```python
from build123d import *

# Parameters (mm, degrees)
SKETCH2_W           = 200
SKETCH2_H           = 150
SKETCH2_W_2         = 190
SKETCH2_H_2         = 140
BOSS_EXTRUDE1_DEPTH = 1800
SKETCH5_R           = 2.5
CUT_EXTRUDE3_DEPTH  = 10
SKETCH6_R           = 5
SKETCH6_R_2         = 2
CUT_EXTRUDE4_DEPTH  = 5


with BuildPart() as part:
    # Sketch2 → Boss-Extrude1 (new body)
    with BuildSketch(Plane.XY):
        Rectangle(SKETCH2_W, SKETCH2_H)
        Rectangle(SKETCH2_W_2, SKETCH2_H_2, mode=Mode.SUBTRACT)
    extrude(amount=BOSS_EXTRUDE1_DEPTH)

    # Sketch5 → Cut-Extrude3 (cut)
    with BuildSketch(Plane(origin=(0, 75, 0), x_dir=(1, 0, 0), z_dir=(0, 1, 0))):
        with Locations((-32.7, -360)):
            Circle(SKETCH5_R)
        with Locations((-32.7, -480)):
            Circle(SKETCH5_R)
        with Locations((-32.7, -600)):
            Circle(SKETCH5_R)
        with Locations((-32.7, -720)):
            Circle(SKETCH5_R)
        with Locations((-32.7, -840)):
            Circle(SKETCH5_R)
        with Locations((-32.7, -960)):
            Circle(SKETCH5_R)
        with Locations((-32.7, -1080)):
            Circle(SKETCH5_R)
        with Locations((-32.7, -1200)):
            Circle(SKETCH5_R)
        with Locations((-32.7, -1320)):
            Circle(SKETCH5_R)
        with Locations((-32.7, -1440)):
            Circle(SKETCH5_R)
    extrude(amount=-CUT_EXTRUDE3_DEPTH, mode=Mode.SUBTRACT)

    # Sketch6 → Cut-Extrude4 (cut)
    with BuildSketch(Plane.XZ.offset(75)):
        with Locations((-50, 1720)):
            Circle(SKETCH6_R)
        with Locations((50, 1720)):
            Circle(SKETCH6_R)
        with Locations((50, 1590)):
            Circle(SKETCH6_R)
        with Locations((-50, 1590)):
            Circle(SKETCH6_R)
        with Locations((50, 1412.5)):
            Circle(SKETCH6_R_2)
        with Locations((50, 1387.5)):
            Circle(SKETCH6_R_2)
        with Locations((50, 1162.5)):
            Circle(SKETCH6_R_2)
        with Locations((50, 1137.5)):
            Circle(SKETCH6_R_2)
        with Locations((50, 912.5)):
            Circle(SKETCH6_R_2)
        with Locations((50, 887.5)):
            Circle(SKETCH6_R_2)
        with Locations((50, 662.5)):
            Circle(SKETCH6_R_2)
        with Locations((50, 637.5)):
            Circle(SKETCH6_R_2)
        with Locations((50, 412.5)):
            Circle(SKETCH6_R_2)
        with Locations((50, 387.5)):
            Circle(SKETCH6_R_2)
        with Locations((-50, 210)):
            Circle(SKETCH6_R)
        with Locations((50, 210)):
            Circle(SKETCH6_R)
        with Locations((50, 80)):
            Circle(SKETCH6_R)
        with Locations((-50, 80)):
            Circle(SKETCH6_R)
    extrude(amount=-CUT_EXTRUDE4_DEPTH, mode=Mode.SUBTRACT)


solid = part.part
```
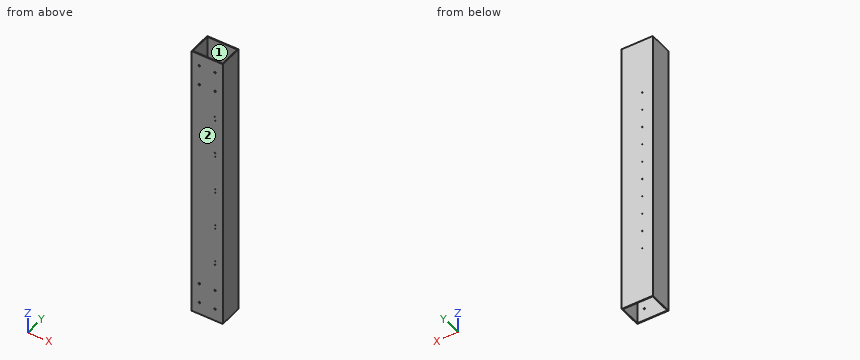
Read the model definition and answer for the solid it produces. Units are mm, in the model's axes. Face numbers are marked on the shaded views. Coordinates: 2 decimals unless noted, no trailing zeros. Order: outer loops, then holes, each group sorted by start corner. A loop starts at its lowest first (then second) coordinate and runs counter-clockwise, first axis right, second up. Notation, with made-up numbers: (70, 47) - (99, 47) arc R20 ccw to (99, 54) - close; hole circle Ø1 at (31, 65). An arc over 180 degrees is marked (long way). Answer as a JSON object with one key per item and string values. Group by question number.
Item 1: Section A-A (y = 11) is taken. Give the vertices of the cut face in (x, z).
Item 2: Section B-B (x = 21.5) is taken. Give the vertices of the cut face in (y, z), plus the area to 3 significant figures.
Item 3: A flat-ended cylindrical pin translates along its axis: P1, Ø2.5, axis at x = 50, z = 662.5, coming from the -Y side. Find the tip coordinate at first contact, or state that the pin passes through.
Item 4: Section C-C (z = 1483.5) is taken. Give the vertices of the cut face in (x, y), plus the area to 3 significant figures.
Item 5: The mould has two halves that part along X. Classify the marked faces 1 and 2: +X half, -X half, draft (parallel to the pull), parting line (faces both ways), or undercut.
Item 6: Consider probe 1 along Y at (x, z) = (-53, 1259.5); probe 2 along X at (y, z) = (62.5, 1700); probe 3 along X at (y, z) = (-73.15, 1137.5). Determine where each line is inside the solid, lowest interval first. Write a range as from..to.
Results are:
{
 "1": {"outline": "(-100, 0) - (-95, 0) - (-95, 1800) - (-100, 1800) - close; (95, 0) - (100, 0) - (100, 1800) - (95, 1800) - close"},
 "2": {"outline": "(-75, 0) - (-70, 0) - (-70, 1800) - (-75, 1800) - close; (70, 0) - (75, 0) - (75, 1800) - (70, 1800) - close", "area": "18,000 mm^2"},
 "3": {"P1": "stops at y = 70"},
 "4": {"outline": "(-100, -75) - (100, -75) - (100, 75) - (-100, 75) - close; hole (-95, -70) - (95, -70) - (95, 70) - (-95, 70) - close", "area": "3,400 mm^2"},
 "5": {"face 1": "undercut", "face 2": "draft"},
 "6": {"probe 1": "y = -75..-70, 70..75", "probe 2": "x = -100..-95, 95..100", "probe 3": "x = -100..48, 52..100"}
}
